from build123d import *

# Parameters (mm, degrees)
F0_W          = 250.825
F0_H          = 76.2
F0_W_2        = 12.7
F0_H_2        = 50.8
F1_DEPTH      = 6.35
F2_DEPTH      = 160.3375
F3_W          = 12.7
F3_H          = 50.8
F4_DEPTH      = 160.3375
F5_W          = 50.8
F5_H          = 12.7
F6_DEPTH      = 152.4
F7_R          = 12.7
F8_DEPTH      = 55.626
F8_DEPTH_BACK = 97.028


with BuildPart() as f1:
    # F0 (on Front) → F1 (new body)
    with BuildSketch(Plane.XZ):
        with Locations((-6.46369, -22.225)):
            Rectangle(F0_W, F0_H)
        with Locations((-103.30119, -25.4)):
            Rectangle(F0_W_2, F0_H_2, mode=Mode.SUBTRACT)
    extrude(amount=F1_DEPTH)

    # F0 (on Front) → F2 (join)
    with BuildSketch(Plane.XZ):
        with Locations((-103.30119, -25.4)):
            Rectangle(F0_W_2, F0_H_2)
    extrude(amount=F2_DEPTH)

    # F3 (on Front) → F4 (join)
    with BuildSketch(Plane.XZ):
        with Locations((54.02811, -19.05)):
            Rectangle(F3_W, F3_H)
    extrude(amount=F4_DEPTH)

    # F5 (on Front) → F6 (join)
    with BuildSketch(Plane.XZ):
        with Locations((85.67481, -23.736117)):
            Rectangle(F5_W, F5_H)
    extrude(amount=F6_DEPTH)

    # F7 (on Right) → F8 (join, two sides)
    with BuildSketch(Plane.YZ) as f8_sk:
        with Locations((-128.5875, -19.05)):
            Circle(F7_R)
    extrude(amount=F8_DEPTH)
    extrude(f8_sk.sketch, amount=-F8_DEPTH_BACK)


solid = f1.part
CAD build for the part. Positions are in the model's coordinates, mm. A direction names the side the tool comes from. Round coordinates to 2 decimals unless told otherwise and drop trailing zeros. Write each loop counter-clockwise with the first axis right and the second up, starting at its lowest first coordinate (ties: lowest second). Pieces come first, ordered by that corner, then holes. Notation, with made-up numbers: (38.5, 0) -> (79.5, 0) arc R22 ccw to (79.5, 17) -> close; hole circle Ø1 at (72, 38.5). An arc over 180 degrees is marked (long way). Answer as a JSON object with one key per item and string values.
(1) Which spindle directions (+Z, -Z, +X, -X, +Y, -Y) get a long thin tool onto all of the face, cutting with end or side? Do faces 5 (the face through (-103, -82, -50.8)), 6 (the face through (-103, -82, 0)), 7 (the face through (-109.651, -82, -26)). Say none if no direction does.
Reported:
{"face 5": "-Z, +X, -X, -Y", "face 6": "+Z, -X, -Y", "face 7": "+Z, -Z, -X, -Y"}
(2) Probe probe 1 along X at (y, z) = (-133.5, -5.5); probe 2 along X at (y, z) = (-65.5, -26); probe 3 along Z at (x, y) = (62, -104.5). List the from-to ranges inside material, lowest first. Write a range as [from, to].
Reported:
{"probe 1": "x = [-109.65, -96.95], [47.68, 60.38]", "probe 2": "x = [-109.65, -96.95], [47.68, 111.07]", "probe 3": "z = [-30.09, -17.39]"}
(3) Band-saw the part on C-C, the plane z = -40. List the corners of the cut face in (x, y).
Reported:
{"outline": "(-131.88, -6.35) -> (-109.65, -6.35) -> (-109.65, -160.34) -> (-96.95, -160.34) -> (-96.95, -6.35) -> (47.68, -6.35) -> (47.68, -160.34) -> (60.38, -160.34) -> (60.38, -6.35) -> (118.95, -6.35) -> (118.95, 0) -> (-131.88, 0) -> close"}
(4) Pin check, flat tips, straight feed: P1, Ø1.5, axis at y = -41.5, z = -45.5, coming from the +X side; P2, Ø14, axis at x = -104.5, y = -72.5, coming from the +Z side; P3, Ø1.5, axis at y = -103, z = -8, coming from the -X side; P4, Ø2, axis at x = 8.5, z = -34, coming from the +Y side. Stop position of each tip, or through.
Reported:
{"P1": "stops at x = -96.95", "P2": "stops at z = 0", "P3": "stops at x = -109.65", "P4": "stops at y = 0"}
(5) Two-plate mould, pull along Y, no slides. Class faces 1 (the face through (-103, -160.338, -25)), 2 (the face through (60.378, -82, -14)), 3 (the face through (-96.951, -82, -26)), 4 (the face through (-8, -6.35, -22)): +Y half, -Y half, draft (parallel to the pull), parting line (faces both ways), or undercut.
Reported:
{"face 1": "-Y half", "face 2": "draft", "face 3": "undercut", "face 4": "undercut"}
(6) Band-saw the part on A-A, the plane y = -70. List the corners of the cut face in (x, z).
Reported:
{"outline": "(-109.65, -50.8) -> (-96.95, -50.8) -> (-96.95, 0) -> (-109.65, 0) -> close; (47.68, -44.45) -> (60.38, -44.45) -> (60.38, -30.09) -> (111.07, -30.09) -> (111.07, -17.39) -> (60.38, -17.39) -> (60.38, 6.35) -> (47.68, 6.35) -> close"}
(7) Band-saw the part on D-D, the plane x = 90. List the corners of the cut face in (y, z) (3 decimals).
Reported:
{"outline": "(-152.4, -30.086) -> (-6.35, -30.086) -> (-6.35, -60.325) -> (0, -60.325) -> (0, 15.875) -> (-6.35, 15.875) -> (-6.35, -17.386) -> (-152.4, -17.386) -> close"}
